Part print with two shaded views. Sizes in mm from the minimum x, y, z corner. A direction names the side the tool comes from. Coordinates: 2 decimals unless noted, no trailing zeros. Loops run counter-clockwise (first coordinate to the right, second up) from the corner with the lowest first, then second, coordinate; pieces in that order, holes last.
Item 1: 3-axis set-ups, long thin cutter, end or side, ignore diameter. For the marked faces 1 and 2: which of +Z, -Z, +X, -X, +Y, -Y reach the whole face in a straight line?
Item 2: Cut at B-B (x = 10). List the corners of the cut face in (y, z), and give its area (3 significant figures).
Item 3: Mould opens along X. For the marked faces 3, 4 and 5 say: released by +X, released by -X, zero draft, split by the parting line, or undercut.
Item 4: Cut at C-C (z = 27.5). List the corners of the cut face in (x, y).
Item 5: Cut at D-D (y = 10). List the corners of the cut face in (x, z).
Item 6: Drill centre lines: line 1 along Y through (x, z) = (10, 19); line 2 along Z through (x, y) = (18.25, 13.25); line 3 along X through (y, z) = (5, 27). Where is each one in solid material? Low to high.
Item 7: Cut at A-A (y = 7.5). List the corners of the cut face in (x, z).
Item 8: Flat gauge pins, fed straight in: pin 1 (3 mm diameter, centred on x = 2.5, z = 22, fed in from -Y); pin 2 (2 mm diameter, centred on x = 12.5, z = 39.5, fed in from +Y); pin 3 (8 mm diameter, centred on x = 10.5, y = 17.5, fed in from -Z); pin 4 (5 mm diameter, centred on x = 3, y = 10.5, fed in from +Z). Where does each tip first touch, or does it go through?
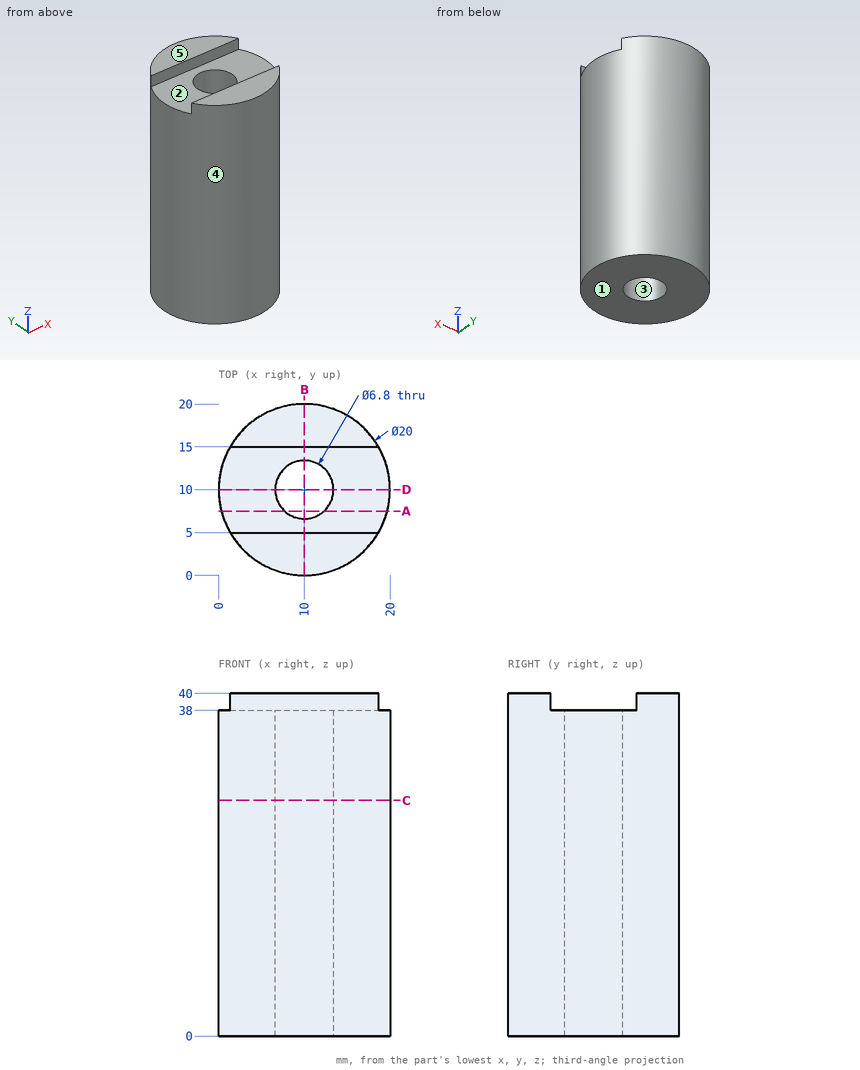
Filled sheet:
1. face 1: -Z, +X, -X, +Y, -Y
1. face 2: +Z, +X, -X
2. outline: (0, 0) - (6.6, 0) - (6.6, 38) - (5, 38) - (5, 40) - (0, 40) - close; (13.4, 0) - (20, 0) - (20, 40) - (15, 40) - (15, 38) - (13.4, 38) - close
2. area: 522 mm2
3. face 3: undercut
3. face 4: split by the parting line
3. face 5: zero draft
4. outline: circle Ø20 at (10, 10); hole circle Ø6.8 at (10, 10)
5. outline: (0, 0) - (6.6, 0) - (6.6, 38) - (0, 38) - close; (13.4, 0) - (20, 0) - (20, 38) - (13.4, 38) - close
6. line 1: y = 0 to 6.6, 13.4 to 20
6. line 2: z = 0 to 38
6. line 3: x = 1.34 to 18.66
7. outline: (0.32, 0) - (7.7, 0) - (7.7, 38) - (0.32, 38) - close; (12.3, 0) - (19.68, 0) - (19.68, 38) - (12.3, 38) - close
8. pin 1: stops at y = 2
8. pin 2: stops at y = 19.89
8. pin 3: stops at z = 0
8. pin 4: stops at z = 38
